Build history of the part. All positions in model axes, mm. Face numbers are marked on the shaded views. A direction names the side the tool comes from. Round coordinates to 2 decimals unless told otherwise and drop trailing zeros. Write each loop counter-clockwise with the first axis right and the second up, starting at its lowest first coordinate (ties: lowest second). Pieces come first, ordered by that corner, then holes.
from build123d import *

# Parameters (mm, degrees)
PAD_DEPTH = 10


with BuildPart() as part:
    # Sketch → Pad (new body)
    with BuildSketch(Plane.XY):
        with BuildLine():
            Line((0, -4), (20, -4))
            Line((20, -4), (20, -7))
            Line((20, -7), (-3, -7))
            Line((-3, -7), (-3, 3))
            Line((-3, 3), (17, 3))
            Line((17, 3), (17, 38))
            Line((17, 38), (93.296024, 59.677571))
            Line((93.296024, 56.677571), (93.296024, 59.677571))
            Line((25.385638, 31.960212), (93.296024, 56.677571))
            ThreePointArc((25.385638, 31.960212), (21.480261, 28.96351), (20, 24.268723))
            Line((20, 0), (20, 24.268723))
            Line((0, 0), (20, 0))
            Line((0, -4), (0, 0))
        make_face()
    extrude(amount=PAD_DEPTH)


solid = part.part
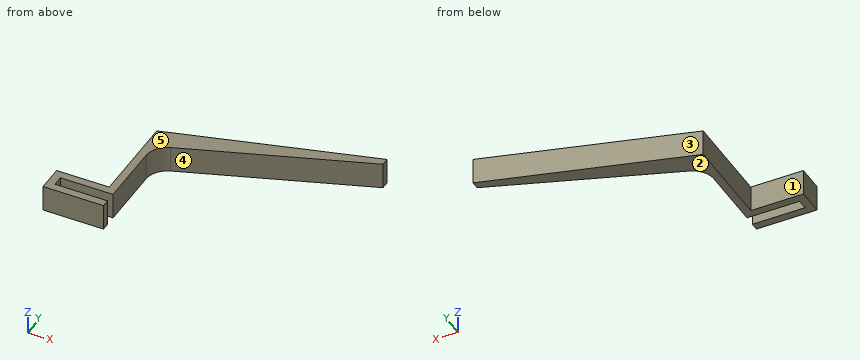
1) Which spindle directions (+Z, -Z, +X, -X, +Y, -Y) get a long thin tool onto all of the face, cutting with end or side? Do the marked faces 1 and 2. Say none if no direction does.
Results:
face 1: +Z, -Z, -X, +Y
face 2: -Z, +X, -X, +Y, -Y
2) Slice it at A-A (x = 5). Write the cut outline in (y, z), plus the area to 3 significant figures.
Results:
outline: (-7, 0) - (-4, 0) - (-4, 10) - (-7, 10) - close; (0, 0) - (3, 0) - (3, 10) - (0, 10) - close
area: 60.0 mm2
3) Pin check, flat tips, straight feed: pin 1 Ø3 at (y, z) = (9.5, 7) entering from +X; pin 2 Ø1.5 at (y, z) = (28, 9) entering from -X; pin 3 Ø2 at (x, z) = (72, 6.5) entering from +Y. Stop position of each tip, or through.
Results:
pin 1: stops at x = 20
pin 2: stops at x = 17
pin 3: stops at y = 53.91
4) Slice it at B-B (z = 9). Write the cut outline in (x, y), plus the area to 3 significant figures.
Results:
outline: (-3, -7) - (20, -7) - (20, -4) - (0, -4) - (0, 0) - (20, 0) - (20, 24.27) arc R8.19 cw to (25.39, 31.96) - (93.3, 56.68) - (93.3, 59.68) - (17, 38) - (17, 3) - (-3, 3) - close
area: 697 mm2
5) Mould opens along Y. For the marked faces 3, 4 and 5 say: released by +Y, released by -Y, zero draft, split by the parting line, or undercut.
Results:
face 3: released by +Y
face 4: released by -Y
face 5: zero draft
6) Slice it at C-C (y = 23). Write the cut outline in (x, z), plus the area to 3 significant figures.
Results:
outline: (17, 0) - (20, 0) - (20, 10) - (17, 10) - close
area: 30.0 mm2
7) Slice it at D-D (x = 52.5). Write the cut outline in (y, z), plus the area to 3 significant figures.
Results:
outline: (41.83, 0) - (48.09, 0) - (48.09, 10) - (41.83, 10) - close
area: 62.6 mm2
8) Wall check: L1, parallel to Y at x = 8, z = 3.5; L2, parallel to X at y = 23.5, z = 4.75; L3, parallel to Y at x = 80.5, z = 2.5. Give the ranges that are in metal, low to high.
Results:
L1: y = -7 to -4, 0 to 3
L2: x = 17 to 20
L3: y = 52.02 to 56.04
